Design review of the part built by this model. Coordinates are the model's own, in mm. Coordinates: 2 decimals unless noted, no trailing zeros. Loops run counter-clockwise (first coordinate to the right, second up) from the corner with the lowest first, then second, coordinate; pieces in that order, holes last. Notation, with made-up numbers: (43, 69) - (58, 69) arc R21 cw to (58, 107) - close; hole circle Ø2 at (-22.75, -25). An arc over 180 degrees is marked (long way). One line per question, with ' | ' between items.
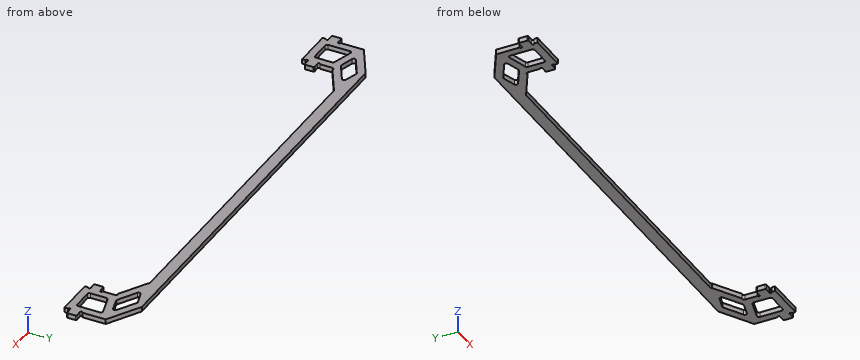
from build123d import *

# Parameters (mm, degrees)
EXTRUDE_1_DEPTH     = 1.25
SKETCH_2_W          = 3.5
SKETCH_2_H          = 5
EXTRUDE_2_DEPTH     = 2.5
SKETCH_3_R          = 0.6
CUT_EXTRUDE_1_DEPTH = 3.5
FILLET_1_R          = 0.5
CUT_EXTRUDE_3_DEPTH = 3.5
CUT_EXTRUDE_5_DEPTH = 3.5
CUT_EXTRUDE_6_DEPTH = 3.5
FILLET_4_R          = 1
SKETCH_12_R         = 1
CUT_EXTRUDE_7_DEPTH = 3.5
SKETCH_13_W         = 157.663481756
SKETCH_13_H         = 52.44668755
CUT_EXTRUDE_8_DEPTH = 3.5


with BuildPart() as part:
    # 草图1 → 凸台-拉伸1 (new body, symmetric)
    with BuildSketch(Plane.XY):
        Polygon((-126.75, 40), (-126.75, 0), (-106.75, 0), (-106.75, 15.5), (-90.295517328, 25), (101.265172443, 25), (106.75, 15.5), (106.75, 0), (126.75, 0), (126.75, 40), align=None)
    extrude(amount=EXTRUDE_1_DEPTH, both=True)

    # 草图2 → 凸台-拉伸2 (add)
    with BuildSketch(Plane.XY.offset(1.25)):
        with Locations((-105, 5.5)):
            Rectangle(SKETCH_2_W, SKETCH_2_H)
        with Locations((105, 5.5)):
            Rectangle(SKETCH_2_W, SKETCH_2_H)
        with Locations((-128.5, 5.5)):
            Rectangle(SKETCH_2_W, SKETCH_2_H)
        with Locations((128.5, 5.5)):
            Rectangle(SKETCH_2_W, SKETCH_2_H)
    extrude(amount=-EXTRUDE_2_DEPTH)

    # 草图3 → 切除-拉伸1 (cut, through all)
    with BuildSketch(Plane.XY.offset(1.25)):
        with Locations((-106.75, 8.6)):
            Circle(SKETCH_3_R)
        with Locations((-106.75, 2.4)):
            Circle(SKETCH_3_R)
        with Locations((106.75, 8.6)):
            Circle(SKETCH_3_R)
        with Locations((106.75, 2.4)):
            Circle(SKETCH_3_R)
        with Locations((-126.75, 8.6)):
            Circle(SKETCH_3_R)
        with Locations((-126.75, 2.4)):
            Circle(SKETCH_3_R)
        with Locations((126.75, 8.6)):
            Circle(SKETCH_3_R)
        with Locations((126.75, 2.4)):
            Circle(SKETCH_3_R)
    extrude(amount=-CUT_EXTRUDE_1_DEPTH, mode=Mode.SUBTRACT)

    # 圆角1
    fillet_1_edges = [part.edges().sort_by_distance(p)[0] for p in [
        (-103.25, 8, 0),
        (-103.25, 3, 0),
        (103.25, 3, 0),
        (103.25, 8, 0),
        (-130.25, 3, 0),
        (-130.25, 8, 0),
        (130.25, 8, 0),
        (130.25, 3, 0),
    ]]
    fillet(fillet_1_edges, radius=FILLET_1_R)

    # 草图7 → 切除-拉伸3 (cut, through all)
    with BuildSketch(Plane.XY.offset(1.25)):
        Polygon((-126.75, 21.273502692), (-94.314755215, 40), (-126.75, 40), align=None)
        Polygon((109.925426481, 40), (126.75, 40), (126.75, 10.858983849), align=None)
    extrude(amount=-CUT_EXTRUDE_3_DEPTH, mode=Mode.SUBTRACT)

    # 草图10 → 切除-拉伸5 (cut, through all)
    with BuildSketch(Plane.XY.offset(1.25)):
        Polygon((-109.903212483, 31), (59.199644147, 31), (69.925426481, 40), (-94.314755215, 40), align=None)
    extrude(amount=-CUT_EXTRUDE_5_DEPTH, mode=Mode.SUBTRACT)

    # 草图11 → 切除-拉伸6 (cut, through all)
    with BuildSketch(Plane.XY.offset(1.25)):
        Polygon((-107.634159118, 27.691236417), (-119.613891029, 20.774734974), (-110.280557696, 18.080433718), (-98.483901379, 24.891236417), align=None)
        Polygon((-122.75, 17.516719654), (-122.75, 4), (-110.75, 4), (-110.75, 14.052618039), align=None)
        Polygon((122.75, 10.247330901), (122.75, 4), (110.75, 4), (110.75, 13.031940592), align=None)
    extrude(amount=-CUT_EXTRUDE_6_DEPTH, mode=Mode.SUBTRACT)

    # 圆角4
    fillet_4_edges = [part.edges().sort_by_distance(p)[0] for p in [
        (-107.634159118, 27.691236417, 0),
        (-98.483901379, 24.891236417, 0),
        (-110.280557696, 18.080433718, 0),
        (-119.613891029, 20.774734974, 0),
        (-110.75, 4, 0),
        (-122.75, 4, 0),
        (-122.75, 17.516719654, 0),
        (-110.75, 14.052618039, 0),
        (122.75, 4, 0),
        (110.75, 4, 0),
        (110.75, 13.031940592, 0),
        (122.75, 10.247330901, 0),
    ]]
    fillet(fillet_4_edges, radius=FILLET_4_R)

    # 草图12 → 切除-拉伸7 (cut, through all)
    with BuildSketch(Plane.XY.offset(1.25)):
        with Locations((-90.295517328, 24)):
            Circle(SKETCH_12_R)
        with Locations((-105.75, 15.5)):
            Circle(SKETCH_12_R)
        with Locations((59.199644147, 32)):
            Circle(SKETCH_12_R)
        with Locations((101.265172443, 24)):
            Circle(SKETCH_12_R)
        with Locations((105.75, 15.5)):
            Circle(SKETCH_12_R)
    extrude(amount=-CUT_EXTRUDE_7_DEPTH, mode=Mode.SUBTRACT)

    # 草图13 → 切除-拉伸8 (cut, through all)
    with BuildSketch(Plane.XY.offset(1.25)):
        with Locations((78.831740878, 26.223343775)):
            Rectangle(SKETCH_13_W, SKETCH_13_H)
    extrude(amount=-CUT_EXTRUDE_8_DEPTH, mode=Mode.SUBTRACT)

    # 镜向2: part across plane


with BuildPart() as part_1:
    add(part.part)
    add(part.part.mirror(Plane(origin=(0, 52.44668755, -1.25), x_dir=(0, 0, 1), z_dir=(-1, 0, 0))))


solid = part_1.part
Q1. For pin 1 (1.2 mm diameter, centred on y = 10.5, z = 0, fed in from +X); pin 2 (1.5 mm diameter, centred on x = -39.5, z = 0.5, fed in from -Y); pin 3 (1.2 mm diameter, centred on x = 115, z = -0.5, fed in from +Y), all flat-tipped, find the tip position at first contact; note any pin that passes through.
Returned:
pin 1: stops at x = 126.75 | pin 2: stops at y = 25 | pin 3: stops at y = 28.4
Q2. To check wall thickness, follow line 1 along X through (y, z) = (7, 0.65); line 2 along X through (y, z) = (12, 0.25); line 3 along Y through (x, z) = (-117, 0.1). State the ranges of each line that lie inside material, in increasing order.
Returned:
line 1: x = -130.25 to -122.75, -110.75 to -103.25, 103.25 to 110.75, 122.75 to 130.25 | line 2: x = -126.75 to -122.75, -110.75 to -106.75, 106.75 to 110.75, 122.75 to 126.75 | line 3: y = 0 to 4, 15.86 to 20.02, 22.28 to 26.9
Q3. Take a section at B-B (x = 25.5). Give the boundary of the cut face in (y, z), plus the area to 3 significant figures.
Returned:
outline: (25, -1.25) - (31, -1.25) - (31, 1.25) - (25, 1.25) - close | area: 15.0 mm²
Q4. Take a section at A-A (z = 0.5). State how many separate pieces and enclosed holes the cut face has, plus the area to 3 significant figures.
Returned:
separate pieces: 1 | enclosed holes: 4 | area: 2,110 mm²
